Check sheet for the modelled part. Datum: model origin and axes. Units: mm. A direction names the side the tool comes from. Give positions to 0.01 mm unless a question says otherwise; leave off trailing zeros. Loops run counter-clockwise (first coordinate to the right, second up) from the corner with the lowest first, then second, coordinate; pieces in that order, holes last. Notation, with made-up numbers: M 37,26 L 66,26 A24 ccw 66,64 Z; hole C -37,88 d10. An arc over 180 degrees is marked long. Use one line per item in the form item = value.
from build123d import *

# Parameters (mm, degrees)
F_1_2_0_5_DIAMETER_HOLE2_D     = 12.7
F_1_2_0_5_DIAMETER_HOLE2_DEPTH = 12.7
F_1_2_0_5_DIAMETER_HOLE2_TIP   = 3.815464931
F_4_40_TAPPED_HOLE1_REACH      = 51.289
F_4_40_TAPPED_HOLE1_BORE_R     = 1.1303
CHAMFER1_SIZE                  = 0.508


with BuildPart() as part:
    # Sketch → Shaft (revolve)
    with BuildSketch(Plane(origin=(0, 0, 0), x_dir=(0, 0, -1), z_dir=(1, 0, 0)), mode=Mode.PRIVATE) as shaft_sk:
        Polygon((0, 0), (0, 3.175), (24.765, 3.175), (24.765, 9.525), (44.45, 9.525), (44.45, 0), align=None)
    revolve(shaft_sk.sketch.rotate(Axis((0, 0, -44.45), (0, 0, 1)), 90), axis=Axis((0, 0, -44.45), (0, 0, 1)))

    # 1/2 (0.5) Diameter Hole2
    with Locations(Plane(origin=(0, 0, -44.45), x_dir=(-1, 0, 0), z_dir=(0, 0, -1))):
        with Locations((0, 0)):
            Hole(F_1_2_0_5_DIAMETER_HOLE2_D / 2, depth=F_1_2_0_5_DIAMETER_HOLE2_DEPTH)
            with Locations((0, 0, -(F_1_2_0_5_DIAMETER_HOLE2_DEPTH + F_1_2_0_5_DIAMETER_HOLE2_TIP / 2))):  # 118° drill point
                Cone(0, F_1_2_0_5_DIAMETER_HOLE2_D / 2, F_1_2_0_5_DIAMETER_HOLE2_TIP, mode=Mode.SUBTRACT)

    # #4-40 Tapped Hole1 bore → #4-40 Tapped Hole1 (cut, up to next)
    with BuildSketch(Plane(origin=(0, -9.525, 0), x_dir=(-1, 0, 0), z_dir=(0, -1, 0)), mode=Mode.PRIVATE) as f_4_40_tapped_hole1_sk1:
        with Locations((0, 34.925)):
            Circle(F_4_40_TAPPED_HOLE1_BORE_R)
    f_4_40_tapped_hole1_tool1 = extrude(f_4_40_tapped_hole1_sk1.sketch, amount=-F_4_40_TAPPED_HOLE1_REACH, mode=Mode.PRIVATE) & part.part
    # #4-40 Tapped Hole1 bore → #4-40 Tapped Hole1 (cut, up to next)
    with BuildSketch(Plane(origin=(0, -9.525, 0), x_dir=(-1, 0, 0), z_dir=(0, -1, 0)), mode=Mode.PRIVATE) as f_4_40_tapped_hole1_sk2:
        with Locations((0, 41.275)):
            Circle(F_4_40_TAPPED_HOLE1_BORE_R)
    f_4_40_tapped_hole1_tool2 = extrude(f_4_40_tapped_hole1_sk2.sketch, amount=-F_4_40_TAPPED_HOLE1_REACH, mode=Mode.PRIVATE) & part.part
    add(f_4_40_tapped_hole1_tool1.solids().sort_by_distance((0, -9.525, -34.925))[0], mode=Mode.SUBTRACT)
    add(f_4_40_tapped_hole1_tool2.solids().sort_by_distance((0, -9.525, -41.275))[0], mode=Mode.SUBTRACT)

    # Chamfer1
    chamfer1_edges = [part.edges().sort_by_distance(p)[0] for p in [
        (-6.35, 0, -44.45),
        (3.175, 0, 0),
    ]]
    chamfer(chamfer1_edges, length=CHAMFER1_SIZE)


solid = part.part
1) Section check C-C (z = -30.5). Record the cut outline in (x, y) (3 decimals), then the cut area to 3 significant figures.
Evaluation:
outline = C 0,0 d19.05; hole C 0,0 d8.539
area = 228 mm^2
2) Scan lines: line 1 (Z direction, x = 0, y = -6.9) (3 decimals); line 2 (X direction, y = 0.25, z = -5); line 3 (X direction, y = -4.5, z = -37.5). Record each from-to range of solid material in increasing order.
Evaluation:
line_1 = -44.45 to -42.405, -40.145 to -36.055, -33.795 to -24.765
line_2 = -3.17 to 3.17
line_3 = -8.39 to -4.48, 4.48 to 8.39
3) Depth check by flat-ended pin: pin 1 Ø2 at (x, y) = (-7, -0.5) entering from +Z (3 decimals); pin 2 Ø1 at (x, y) = (2.5, -5.5) entering from -Z; pin 3 Ø2.5 at (x, z) = (0, -41.275) entering from -Y (3 decimals); pin 4 Ø3 at (y, z) = (7, -38) entering from -X. Enter the tip coordinate at first touch or a pass-through.
Evaluation:
pin_1 = -24.765
pin_2 = -44.13
pin_3 = -9.525
pin_4 = -7.78
4) Set-up check for faces 4 (the face through (0.245, -7.908, -40.172)), 5 (the face through (4, 0, -24.765)), 6 (the face through (0.88, -0.67, -28.6)): record each of +Z, -Z, +X, -X, +Y, -Y from which the full face is reachable in a straight line by a thin tool's end or side.
Evaluation:
face_4 = -Y
face_5 = +Z
face_6 = -Z
5) Section check B-B (z = -19). Record the cut outline in (x, y) (3 decimals).
Evaluation:
outline = C 0,0 d6.35
6) Section check A-A (x = -0.5). State how many separate pieces and enclosed holes the cut face has, then the cut area to 3 significant figures.
Evaluation:
separate_pieces = 3
enclosed_holes = 0
area = 332 mm^2
7) Release check for a two-part mould opening along X. For faces 1 (the face through (-1.38, -6.2, -37.76)), 2 (the face through (0, 0, 0)), 3 (the face through (2.06, 9.3, -34.75)) record: pulls with the +X half, pulls with the -X half, needs draft (parallel to the pull), parting line crosses it, or undercut.
Evaluation:
face_1 = undercut
face_2 = needs draft
face_3 = parting line crosses it
8) Section check D-D (y = 8.25). Record the cut outline in (x, z) (3 decimals).
Evaluation:
outline = M -4.761,-44.45 L 4.761,-44.45 L 4.761,-24.765 L -4.761,-24.765 Z
